```python
from build123d import *

# Parameters (mm, degrees)
SKETCH1_R           = 10
BOSS_EXTRUDE1_DEPTH = 6
SKETCH2_R           = 0.75
CUT_EXTRUDE1_DEPTH  = 15
SKETCH4_R           = 6
BOSS_EXTRUDE3_DEPTH = 10
SKETCH5_W           = 20
SKETCH5_H           = 20
BOSS_EXTRUDE4_DEPTH = 4.5
BOSS_EXTRUDE5_DEPTH = 9
SKETCH7_W           = 15
SKETCH7_H           = 35
CUT_EXTRUDE2_DEPTH  = 4
CUT_EXTRUDE3_DEPTH  = 14
CUT_EXTRUDE4_DEPTH  = 10
SKETCH11_R          = 1.95
SKETCH11_R_2        = 1.5
BOSS_EXTRUDE6_DEPTH = 3.5
SKETCH12_R          = 3
BOSS_EXTRUDE7_DEPTH = 3.5
SKETCH13_R          = 1.5
CUT_EXTRUDE5_DEPTH  = 25
FILLET1_R           = 20
FILLET2_R           = 10
FILLET3_R           = 3
FILLET4_R           = 3
FILLET5_R           = 3
FILLET6_R           = 3


with BuildPart() as part:
    # Sketch1 → Boss-Extrude1 (new body)
    with BuildSketch(Plane.XY):
        Circle(SKETCH1_R)
    extrude(amount=BOSS_EXTRUDE1_DEPTH)

    # Sketch2 → Cut-Extrude1 (cut)
    with BuildSketch(Plane.XY.offset(6)):
        with Locations((0, 7.25)):
            Circle(SKETCH2_R)
        with Locations((4, 7.25)):
            Circle(SKETCH2_R)
        with Locations((-4, 7.25)):
            Circle(SKETCH2_R)
        with Locations((4, -7.25)):
            Circle(SKETCH2_R)
        with Locations((0, -7.25)):
            Circle(SKETCH2_R)
        with Locations((-4, -7.25)):
            Circle(SKETCH2_R)
    extrude(amount=-CUT_EXTRUDE1_DEPTH, mode=Mode.SUBTRACT)

    # Sketch4 → Boss-Extrude3 (add)
    with BuildSketch(Plane(origin=(0, 0, 0), x_dir=(-1, 0, 0), z_dir=(0, 0, -1))):
        Circle(SKETCH4_R)
    extrude(amount=BOSS_EXTRUDE3_DEPTH)

    # Sketch5 → Boss-Extrude4 (add, symmetric)
    with BuildSketch(Plane(origin=(0, 0, 0), x_dir=(1, 0, 0), z_dir=(0, 1, 0))):
        with Locations((0, 10)):
            Rectangle(SKETCH5_W, SKETCH5_H)
    extrude(amount=BOSS_EXTRUDE4_DEPTH, both=True)

    # Sketch6 → Boss-Extrude5 (add)
    with BuildSketch(Plane(origin=(0, 4.5, 0), x_dir=(1, 0, 0), z_dir=(0, 1, 0))):
        Polygon((10, 20), (35.763212592, 40.556396064), (35.763212592, 98.883063355), (-35.763212592, 98.883063355), (-35.763212592, 40.556396064), (-10, 20), align=None)
    extrude(amount=-BOSS_EXTRUDE5_DEPTH)

    # Sketch7 → Cut-Extrude2 (cut)
    with BuildSketch(Plane.XZ.offset(4.5)):
        with Locations((-11.892304399, -51.30711123)):
            Rectangle(SKETCH7_W, SKETCH7_H)
    extrude(amount=-CUT_EXTRUDE2_DEPTH, mode=Mode.SUBTRACT)

    # Sketch8 → Cut-Extrude3 (cut)
    with BuildSketch(Plane.XZ.offset(0.5)):
        Polygon((-18.192304399, -55.774359721), (-18.192304399, -40.505749007), (-5.592304399, -40.505749007), (-5.592304399, -55.774359721), (-5.592304399, -64.974058921), (-18.192304399, -64.974058921), align=None)
    extrude(amount=-CUT_EXTRUDE3_DEPTH, mode=Mode.SUBTRACT)

    # Sketch10 → Cut-Extrude4 (cut)
    with BuildSketch(Plane.XZ.offset(4.5)):
        Polygon((-21.939786422, -73.769938093), (-14.445366372, -98.883063355), (-35.763212592, -98.883063355), (-35.763212592, -40.556396064), (-21.939786422, -29.526722559), align=None)
        Polygon((35.763212592, -40.556396064), (35.763212592, -98.883063355), (14.445366372, -98.883063355), (21.939786422, -73.769938093), (21.939786422, -29.526722559), align=None)
    extrude(amount=-CUT_EXTRUDE4_DEPTH, mode=Mode.SUBTRACT)

    # Sketch11 → Boss-Extrude6 (add)
    # profile 1 of 2: a face of its own
    with BuildSketch(Plane(origin=(0, 4.5, 0), x_dir=(1, 0, 0), z_dir=(0, 1, 0))):
        with Locations(Location((-11.689786422, 87.703063355, 0), (0, 0, 270))):
            Circle(SKETCH11_R)
        with Locations(Location((-11.689786422, 87.703063355, 0), (0, 0, 270))):
            Circle(SKETCH11_R_2, mode=Mode.SUBTRACT)
    # profile 2 of 2: a face of its own
    with BuildSketch(Plane(origin=(0, 4.5, 0), x_dir=(1, 0, 0), z_dir=(0, 1, 0))):
        with Locations(Location((7.610213578, 87.703063355, 0), (0, 0, 270))):
            Circle(SKETCH11_R)
        with Locations(Location((7.610213578, 87.703063355, 0), (0, 0, 270))):
            Circle(SKETCH11_R_2, mode=Mode.SUBTRACT)
    extrude(amount=BOSS_EXTRUDE6_DEPTH)

    # Sketch12 → Boss-Extrude7 (add)
    with BuildSketch(Plane(origin=(0, 4.5, 0), x_dir=(1, 0, 0), z_dir=(0, 1, 0))):
        with Locations(Location((7.610213578, 47.703063355, 0), (0, 0, 270))):
            Circle(SKETCH12_R)
    extrude(amount=BOSS_EXTRUDE7_DEPTH)

    # Sketch13 → Cut-Extrude5 (cut)
    with BuildSketch(Plane(origin=(0, 8, 0), x_dir=(1, 0, 0), z_dir=(0, 1, 0))):
        with Locations(Location((7.610213578, 47.703063355, 0), (0, 0, 270))):
            Circle(SKETCH13_R)
    extrude(amount=-CUT_EXTRUDE5_DEPTH, mode=Mode.SUBTRACT)

    # Fillet1
    fillet1_edges = [part.edges().sort_by_distance(p)[0] for p in [
        (10, 0, -20),
        (-10, 0, -20),
    ]]
    fillet(fillet1_edges, radius=FILLET1_R)

    # Fillet2
    fillet2_edges = [part.edges().sort_by_distance(p)[0] for p in [
        (-21.939786422, 0, -29.526722559),
        (-21.939786422, 0, -73.769938093),
        (-14.445366372, 0, -98.883063355),
        (21.939786422, 0, -29.526722559),
        (14.445366372, 0, -98.883063355),
        (21.939786422, 0, -73.769938093),
    ]]
    fillet(fillet2_edges, radius=FILLET2_R)

    # Fillet3
    # the kernel refuses this fillet: 3 mm, written as the material it adds along each edge
    with BuildSketch(Plane(origin=(11.468626967, 4.5, -10), x_dir=(0, 0, -1), z_dir=(-1, 0, 0))) as fillet3_piece_1_section:
        with BuildLine():
            CenterArc((FILLET3_R, -FILLET3_R), FILLET3_R, 90, 90)
            Line((0, -FILLET3_R), (0, 0))
            Line((0, 0), (FILLET3_R, 0))
        make_face()
    fillet3_piece_1 = extrude(amount=22.937253933, mode=Mode.PRIVATE)
    fillet3_piece_1 = fillet3_piece_1 & Plane(origin=(0, 0, -10.801783603), x_dir=(-1, 0, 0), z_dir=(0, 0, 1)) * Cylinder(6, 58, mode=Mode.PRIVATE)
    add(fillet3_piece_1)
    with BuildSketch(Plane(origin=(11.468626967, -4.5, -10), x_dir=(0, 0, -1), z_dir=(-1, 0, 0))) as fillet3_piece_2_section:
        with BuildLine():
            CenterArc((FILLET3_R, FILLET3_R), FILLET3_R, 180, 90)
            Line((0, FILLET3_R), (0, 0))
            Line((0, 0), (FILLET3_R, 0))
        make_face()
    fillet3_piece_2 = extrude(amount=22.937253933, mode=Mode.PRIVATE)
    fillet3_piece_2 = fillet3_piece_2 & Plane(origin=(0, 0, -10.801783603), x_dir=(-1, 0, 0), z_dir=(0, 0, 1)) * Cylinder(6, 58, mode=Mode.PRIVATE)
    add(fillet3_piece_2)

    # Fillet4
    fillet4_edges = [part.edges().sort_by_distance(p)[0] for p in [
        (3.968626967, 4.5, -6.5),
    ]]
    fillet(fillet4_edges, radius=FILLET4_R)

    # Fillet5
    fillet5_edges = [part.edges().sort_by_distance(p)[0] for p in [
        (-3.968626967, 4.5, -6.5),
    ]]
    fillet(fillet5_edges, radius=FILLET5_R)

    # Fillet6
    fillet6_edges = [part.edges().sort_by_distance(p)[0] for p in [
        (-3.968626967, -4.5, -6.5),
        (3.968626967, -4.5, -6.5),
    ]]
    fillet(fillet6_edges, radius=FILLET6_R)


solid = part.part
```
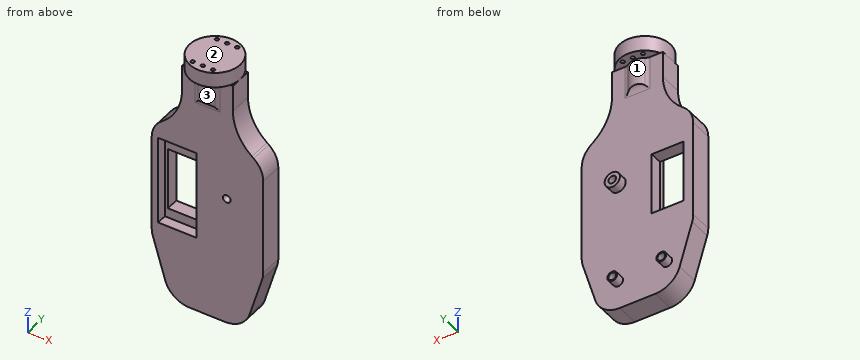
CAD build for the part. Positions are in the model's coordinates, mm. Face numbers are marked on the shaded views. A direction names the side the tool comes from. Give positions to 0.01 mm unless a question says otherwise; leave off trailing zeros. Loops run counter-clockwise (first coordinate to the right, second up) from the corner with the lowest first, then second, coordinate; pieces in that order, holes last. Notation, with made-up numbers: M 76.5,38.25 L 135.5,38.25 A27 ccw 135.5,73.25 Z; hole C -39.5,50.5 d3. An arc over 180 degrees is marked long. Use one line per item in the form item = value.
Item 1: Flat gauge pins, fed straight in: pin 1 (16.5 mm diameter, centred on x = -11.5, z = -49.5, fed in from -Y); pin 2 (10 mm diameter, centred on y = 2, z = -3.5, fed in from +X); pin 3 (12 mm diameter, centred on x = 13, y = -6, fed in from +Z); pin 4 (1.2 mm diameter, centred on x = -12, z = -87.5, fed in from +Y). Where does each tip first touch, or does it go through?
Determined:
pin_1 = -4.5
pin_2 = 10
pin_3 = 6
pin_4 = 4.5
Item 2: Slice it at C-C (x = -8). List the corners of the cut face in (y, z).
Determined:
outline = M -6,0 L -4.5,0 L -4.5,-33.81 L -0.5,-33.81 L -0.5,-40.51 L 4.5,-40.51 L 4.5,0 L 6,0 L 6,6 L -6,6 Z; M -4.5,-98.83 L 4.5,-98.83 L 4.5,-64.97 L -0.5,-64.97 L -0.5,-68.81 L -4.5,-68.81 Z
Item 3: Which spindle directions (+Z, -Z, +X, -X, +Y, -Y) get a long thin tool onto all of the face, cutting with end or side? Do the marked faces 1, 2 and 3. Say none if no direction does.
Determined:
face_1 = -Z, +Y
face_2 = +Z, +X, -X, +Y, -Y
face_3 = -Z, -Y
Item 4: Drill centre lines: probe 1 along Y at (x, z) = (0, 4.3); probe 2 along Z at (x, y) = (-5.5, -3.75); probe 3 along X at (y, z) = (2.5, -61). Where is each one in solid material? Low to high. Write a range as from..to.
Determined:
probe_1 = -10..-8, -6.5..6.5, 8..10
probe_2 = -98.88..-68.81, -33.81..6
probe_3 = -21.94..-18.19, -5.59..21.94
Item 5: Slice it at B-B (y = 2). List the corners of the cut face in (x, z), plus the area to 3 significant figures.
Determined:
outline = M -21.94,-72.31 A10 ccw -21.52,-75.17 L -16.58,-91.74 A10 ccw -6.99,-98.88 L 6.99,-98.88 A10 ccw 16.58,-91.74 L 21.52,-75.17 A10 ccw 21.94,-72.31 L 21.94,-34.34 A10 ccw 18.18,-26.52 L 17.53,-26.01 A20 cw 10,-10.37 L 10,0 L 9.8,0 L 9.8,6 L -9.8,6 L -9.8,0 L -10,0 L -10,-10.37 A20 cw -17.53,-26.01 L -18.18,-26.52 A10 ccw -21.94,-34.34 Z; hole M -18.19,-64.97 L -5.59,-64.97 L -5.59,-40.51 L -18.19,-40.51 Z; hole C 7.61,-47.7 d3
area = 3,360 mm2
Item 6: Slice it at A-A (z = -62). List the corners of the cut face in (x, y).
Determined:
outline = M -21.94,-4.5 L -19.39,-4.5 L -19.39,-0.5 L -18.19,-0.5 L -18.19,4.5 L -21.94,4.5 Z; M -5.59,-0.5 L -4.39,-0.5 L -4.39,-4.5 L 21.94,-4.5 L 21.94,4.5 L -5.59,4.5 Z
Item 7: Slice it at D-D (z = -29). List the corners of the cut face in (x, y), plus the area to 3 significant figures.
Determined:
outline = M -20.39,-4.5 L 20.39,-4.5 L 20.39,4.5 L -20.39,4.5 Z
area = 367 mm2
